from build123d import *

# Parameters (mm, degrees)
BASE_FLANGE1_DEPTH    = 3.175
SKETCH7_W             = 3.302
SKETCH7_H             = 12.7
CUT_EXTRUDE1_DEPTH    = 326.126156068
SKETCH12_W            = 3.175
SKETCH12_H            = 25.4
TAB1_DEPTH            = 3.175
CUT_EXTRUDE2_DEPTH    = 326.126156068
FILLET1_R             = 2.54
CUT_EXTRUDE3_DEPTH    = 316.848888055
FILLET2_R             = 12.7
FILLET3_R             = 2.54
F_6_CLEARANCE_HOLE1_D = 3.7973


# Sheet-metal steps are written as plain solids
with BuildPart() as part:
    # Sketch1 → Base-Flange1 (new body)
    with BuildSketch(Plane(origin=(0, 0, 0), x_dir=(1, 0, 0), z_dir=(0, 1, 0))):
        Polygon((-76.2, 0), (76.2, 0), (76.2, -220.278764113), (113.110108895, -299.432748076), (101.6, -304.8), (63.5, -223.094286329), (63.5, -25.4), (-63.5, -25.4), (-63.5, -223.094286329), (-101.6, -304.8), (-113.110108895, -299.432748076), (-76.2, -220.278764113), align=None)
    extrude(amount=-BASE_FLANGE1_DEPTH)

    # Sketch7 → Cut-Extrude1 (cut, through all)
    with BuildSketch(Plane(origin=(0, 0, 0), x_dir=(1, 0, 0), z_dir=(0, 1, 0))):
        with Locations((-17.78, -6.35)):
            Rectangle(SKETCH7_W, SKETCH7_H)
        with Locations((17.78, -6.35)):
            Rectangle(SKETCH7_W, SKETCH7_H)
    extrude(amount=-CUT_EXTRUDE1_DEPTH, mode=Mode.SUBTRACT)

    # Sketch12 → Tab1 (add)
    with BuildSketch(Plane(origin=(0, 0, 0), x_dir=(1, 0, 0), z_dir=(0, 1, 0))):
        with Locations((-61.9125, -88.9)):
            Rectangle(SKETCH12_W, SKETCH12_H)
        Polygon((-80.130992304, -258.759564419), (-90.865496152, -281.779782209), (-87.987968928, -283.12159519), (-77.25346508, -260.1013774), align=None)
        with Locations((-61.9125, -165.1)):
            Rectangle(SKETCH12_W, SKETCH12_H)
        Polygon((77.25346508, -260.1013774), (87.987968928, -283.12159519), (90.865496152, -281.779782209), (80.130992304, -258.759564419), align=None)
        with Locations((61.9125, -165.1)):
            Rectangle(SKETCH12_W, SKETCH12_H)
        with Locations((61.9125, -88.9)):
            Rectangle(SKETCH12_W, SKETCH12_H)
    extrude(amount=-TAB1_DEPTH)

    # Sketch13 → Cut-Extrude2 (cut, through all)
    with BuildSketch(Plane(origin=(0, 0, 0), x_dir=(1, 0, 0), z_dir=(0, 1, 0))):
        Polygon((-101.6, -304.8), (-98.916374038, -299.044945552), (-101.6, -274.749239894), (-113.110108895, -299.432748076), align=None)
        Polygon((101.6, -304.8), (98.916374038, -299.044945552), (101.6, -274.749239894), (113.110108895, -299.432748076), align=None)
    extrude(amount=-CUT_EXTRUDE2_DEPTH, mode=Mode.SUBTRACT)

    # Fillet1
    fillet1_edges = [part.edges().sort_by_distance(p)[0] for p in [
        (63.5, -1.5875, 152.4),
        (63.5, -1.5875, 177.8),
        (80.130992304, -1.5875, 258.759564419),
        (90.865496152, -1.5875, 281.779782209),
        (-80.130992304, -1.5875, 258.759564419),
        (-90.865496152, -1.5875, 281.779782209),
        (-63.5, -1.5875, 177.8),
        (-63.5, -1.5875, 152.4),
        (-63.5, -1.5875, 101.6),
        (-63.5, -1.5875, 76.2),
        (63.5, -1.5875, 25.4),
        (-63.5, -1.5875, 25.4),
        (63.5, -1.5875, 76.2),
        (63.5, -1.5875, 101.6),
    ]]
    fillet(fillet1_edges, radius=FILLET1_R)

    # Sketch14 → Cut-Extrude3 (cut, through all)
    with BuildSketch(Plane(origin=(0, 0, 0), x_dir=(1, 0, 0), z_dir=(0, 1, 0))):
        with BuildLine():
            Line((-20.927228778, -9.663103241), (-19.431, -8.799255153))
            Line((-19.431, -8.799255153), (-19.431, -9.487125897))
            ThreePointArc((-19.431, -9.487125897), (-19.752208028, -13.204840809), (-20.927228778, -9.663103241))
        make_face()
        with BuildLine():
            Line((-16.129, -8.799255153), (-16.129, -9.487125897))
            ThreePointArc((-16.129, -9.487125897), (-15.807791972, -13.204840809), (-14.632771222, -9.663103241))
            Line((-14.632771222, -9.663103241), (-16.129, -8.799255153))
        make_face()
        with BuildLine():
            Line((19.431, -8.799255153), (19.431, -9.487125897))
            ThreePointArc((19.431, -9.487125897), (19.752208028, -13.204840809), (20.927228778, -9.663103241))
            Line((20.927228778, -9.663103241), (19.431, -8.799255153))
        make_face()
        with BuildLine():
            Line((14.632771222, -9.663103241), (16.129, -8.799255153))
            Line((16.129, -8.799255153), (16.129, -9.487125897))
            ThreePointArc((16.129, -9.487125897), (15.807791972, -13.204840809), (14.632771222, -9.663103241))
        make_face()
    extrude(amount=-CUT_EXTRUDE3_DEPTH, mode=Mode.SUBTRACT)

    # Fillet2
    fillet2_edges = [part.edges().sort_by_distance(p)[0] for p in [
        (76.2, -1.5875, 220.278764113),
        (63.5, -1.5875, 223.094286329),
        (-63.5, -1.5875, 223.094286329),
        (-76.2, -1.5875, 220.278764113),
        (-76.2, -1.5875, 0),
        (76.2, -1.5875, 0),
    ]]
    fillet(fillet2_edges, radius=FILLET2_R)

    # Fillet3
    fillet3_edges = [part.edges().sort_by_distance(p)[0] for p in [
        (-98.916374038, -1.5875, 299.044945552),
        (98.916374038, -1.5875, 299.044945552),
    ]]
    fillet(fillet3_edges, radius=FILLET3_R)

    # #6 Clearance Hole1 (through all)
    with Locations(Plane(origin=(0, 0, 0), x_dir=(1, 0, 0), z_dir=(0, 1, 0))):
        with Locations((69.85, -66.675), (69.85, -111.125), (-69.85, -111.125), (-69.85, -66.675)):
            Hole(F_6_CLEARANCE_HOLE1_D / 2)


solid = part.part
Source: CAD feature listing. Evaluate the final solid. Frame: model axes, mm. A direction names the side the tool comes from. Round coordinates to 2 decimals unless told otherwise and drop trailing zeros. Loops run counter-clockwise (first coordinate to the right, second up) from the corner with the lowest first, then second, coordinate; pieces in that order, holes last.
Q1. Section B-B, the plane z = 188.5. Return loops of the section in (x, y) (3 decimals).
Q2. Section D-D, the plane x = -46. Return loops of the section in (y, z) (3 decimals).
Q3. Access query for faces 5 (the face through (-72.38, -1.61, 3.62)), 6 (the face through (82.546, -1.565, 271.45)). Directions: +Z, -Z, +X, -X, +Y, -Y. A direction counts if a zero-diameter tool reaches every point of the face in a straight line with its end or side. Return the directions, or none.
Q4. Section A-A, the plane z = 84.5. Return loops of the section in (x, y) (3 decimals), plus the area to 3 significant figures.
Q5. Ray query, line 1 (X direction, y = -0.15, z = 149); line 2 (Z direction, x = 69.85, y = -2.25); line 3 (Z direction, x = 51.5, y = -0.9). Return the intervals inside material, ascending.
Q6. Mould query, pull axis X, two halves, no side actions, for faces 1 (the face through (-82.696, -1.565, 271.773)), 2 (the face through (61, -3.175, 81)), 3 (the face through (-89.664, -1.565, 249.153)), 4 (the face through (72.58, -1.61, 3.82)). Classes: pulls with the +X half, pulls with the -X half, needs draft (parallel to the pull), parting line crosses it, or undercut.
Q7. First-contact query: P1, Ø1, axis at y = -1.5, z = 5.5, coming from the +X side; P2, Ø1.6, axis at y = -1.5, z = 126.5, coming from the -X side; P3, Ø1, axis at x = -25.5, y = -0.5, coming from the +Z side. Flat tips, straight axial feed; report the tip coordinate or a pass-through.
Q8. Section C-C, the plane z = 20.5. Return loops of the section in (x, y) (3 decimals).
Solutions:
1. outline: (-76.2, -3.175) - (-63.5, -3.175) - (-63.5, 0) - (-76.2, 0) - close; (63.5, -3.175) - (76.2, -3.175) - (76.2, 0) - (63.5, 0) - close
2. outline: (-3.175, 0) - (0, 0) - (0, 25.4) - (-3.175, 25.4) - close
3. face 5: -Z, -X, +Y, -Y
3. face 6: +Z, +Y, -Y
4. outline: (-76.2, -3.175) - (-60.325, -3.175) - (-60.325, 0) - (-76.2, 0) - close; (60.325, -3.175) - (76.2, -3.175) - (76.2, 0) - (60.325, 0) - close
4. area: 101 mm2
5. line 1: x = -76.2 to -63.5, 63.5 to 76.2
5. line 2: z = 1.7 to 64.78, 68.57 to 109.23, 113.02 to 236.71
5. line 3: z = 0 to 25.4
6. face 1: undercut
6. face 2: needs draft
6. face 3: pulls with the -X half
6. face 4: pulls with the +X half
7. P1: stops at x = 74.29
7. P2: stops at x = -76.2
7. P3: stops at z = 25.4
8. outline: (-76.2, -3.175) - (76.2, -3.175) - (76.2, 0) - (-76.2, 0) - close
